from build123d import *

# Parameters (mm, degrees)
SKETCH1_R           = 69.85
BOSS_EXTRUDE1_DEPTH = 6.35
SKETCH4_R           = 0.59055
CUT_EXTRUDE1_DEPTH  = 49.26
CUT_EXTRUDE2_START  = -51.8
SKETCH6_R           = 0.59055
CUT_EXTRUDE2_DEPTH  = 77.349261314
LOX_START           = -7.35
SKETCH7_R           = 0.8255
LOX_HOLES_DEPTH     = 8.35
CIRPATTERN1_COUNT   = 18
SKETCH8_R           = 3.2639
CUT_EXTRUDE4_DEPTH  = 7.35
CIRPATTERN2_COUNT   = 12


with BuildPart() as part:
    # Sketch1 → Boss-Extrude1 (new body)
    with BuildSketch(Plane(origin=(0, 0, 0), x_dir=(1, 0, 0), z_dir=(0, 1, 0))):
        Circle(SKETCH1_R)
    extrude(amount=BOSS_EXTRUDE1_DEPTH)

    # Sketch4 → Cut-Extrude1 (cut, through all)
    with BuildSketch(Plane(origin=(-3.917869343, -6.785948759, 0), x_dir=(-0.866025404, 0.5, 0), z_dir=(0.5, 0.866025404, 0))):
        with Locations((-4.52396584, 0)):
            Circle(SKETCH4_R)
    cut_extrude1 = extrude(amount=CUT_EXTRUDE1_DEPTH, mode=Mode.SUBTRACT)

    # Sketch6 → Cut-Extrude2 (cut)
    with BuildSketch(Plane(origin=(5.187869343, -8.985653285, 0), x_dir=(0.866025404, 0.5, 0), z_dir=(0.5, -0.866025404, 0)).offset(CUT_EXTRUDE2_START)):
        with Locations((30.67130657, 0)):
            Circle(SKETCH6_R)
    cut_extrude2 = extrude(amount=CUT_EXTRUDE2_DEPTH, mode=Mode.SUBTRACT)

    # Sketch7 → LOx Holes (cut)
    with BuildSketch(Plane(origin=(0, 6.35, 0), x_dir=(1, 0, 0), z_dir=(0, 1, 0)).offset(LOX_START)):
        with Locations((24.13, 0)):
            Circle(SKETCH7_R)
        with Locations((16.51, 0)):
            Circle(SKETCH7_R)
    lox_holes = extrude(amount=LOX_HOLES_DEPTH, mode=Mode.SUBTRACT)

    # CirPattern1: Cut-Extrude1, Cut-Extrude2, LOx Holes ×18 about axis
    cirpattern1_axis = Axis((0, 0, 0), (0, 1, 0))
    for i in range(1, CIRPATTERN1_COUNT):
        add(cut_extrude1.rotate(cirpattern1_axis, i * 360 / CIRPATTERN1_COUNT), mode=Mode.SUBTRACT)
        add(cut_extrude2.rotate(cirpattern1_axis, i * 360 / CIRPATTERN1_COUNT), mode=Mode.SUBTRACT)
        add(lox_holes.rotate(cirpattern1_axis, i * 360 / CIRPATTERN1_COUNT), mode=Mode.SUBTRACT)

    # Sketch8 → Cut-Extrude4 (cut, through all)
    with BuildSketch(Plane.XZ):
        with Locations((-60.96, 0)):
            Circle(SKETCH8_R)
    cut_extrude4 = extrude(amount=-CUT_EXTRUDE4_DEPTH, mode=Mode.SUBTRACT)

    # CirPattern2: Cut-Extrude4 ×12 about axis
    cirpattern2_axis = Axis((0, 0, 0), (0, 1, 0))
    for i in range(1, CIRPATTERN2_COUNT):
        add(cut_extrude4.rotate(cirpattern2_axis, i * 360 / CIRPATTERN2_COUNT), mode=Mode.SUBTRACT)


solid = part.part
Build history of the part. All positions in model axes, mm. Coordinates: 2 decimals unless noted, no trailing zeros. Order: outer loops, then holes, each group sorted by start corner. A loop starts at its lowest first (then second) coordinate and runs counter-clockwise, first axis right, second up. Notation, with made-up numbers: (79.25, -28.75) - (129.25, -28.75) arc R20 ccw to (129.25, 7.25) - close; hole circle Ø4 at (46, 1.5). An arc over 180 degrees is marked (long way). Put each result on its own line as item: value.
1. Saw through at A-A (z = -60.96). Write the cut outline in (x, y).
Answer sheet:
outline: (-34.1, 0) - (-3.26, 0) - (-3.26, 6.35) - (-34.1, 6.35) - close; (3.26, 0) - (34.1, 0) - (34.1, 6.35) - (3.26, 6.35) - close
2. Pull direction Y, two halves, no side cores. Call faces 1 (the face through (-5.065, 3.102, -5.014)), 2 (the face through (-16.5, 2.94, -28.62)), 3 (the face through (-30.055, 3.131, 49.557)): pulls with the +Y half, pulls with the -Y half, needs draft (parallel to the pull), parting line crosses it, or undercut.
Answer sheet:
face 1: undercut
face 2: undercut
face 3: needs draft
3. Saw through at C-C (z = 53). Write the cut outline in (x, y), and give its area (3 significant figures).
Answer sheet:
outline: (-45.5, 0) - (-33.74, 0) - (-33.74, 6.35) - (-45.5, 6.35) - close; (-27.22, 0) - (27.22, 0) - (27.22, 6.35) - (-27.22, 6.35) - close; (33.74, 0) - (45.5, 0) - (45.5, 6.35) - (33.74, 6.35) - close
area: 495 mm^2
4. Saw through at D-D (y = 3). Give the number of separate pieces and of enclosed holes in the cut face, and give its area (3 significant figures).
Answer sheet:
separate pieces: 1
enclosed holes: 84
area: 14,800 mm^2
5. Drop flat-ended pins along their axis: P1, Ø3, axis at y = 3.5, z = 31.5, coming from the +X side; P2, Ø3, axis at x = -46.5, y = 4, coming from the -Z side; P3, Ø1, axis at y = 2, z = -11.5, coming from the +X side. Give the stop position or say it passes through.
Answer sheet:
P1: stops at x = 63.08
P2: stops at z = -53.42
P3: stops at x = 68.98
6. Probe line 1 along X through (y, z) = (4.5, -8.5); line 2 along Z through (x, y) = (-18, 1.5); line 3 along X through (y, z) = (5.5, 21). List the from-to ranges inside material, lowest first. Write a range as [from, to].
Answer sheet:
line 1: x = [-69.33, -23.46], [-21.89, 21.89], [23.46, 69.33]
line 2: z = [-67.49, -16.18], [-14.84, 14.84], [16.18, 67.49]
line 3: x = [-66.62, -25.31], [-24.16, -12.88], [-11.25, 11.25], [12.88, 24.16], [25.31, 66.62]
7. Saw through at B-B (x = 53.5). Write the cut outline in (y, z), and give its area (3 significant figures).
Answer sheet:
outline: (0, -44.91) - (6.35, -44.91) - (6.35, -33.67) - (0, -33.67) - close; (0, -27.29) - (6.35, -27.29) - (6.35, 27.29) - (0, 27.29) - close; (0, 33.67) - (6.35, 33.67) - (6.35, 44.91) - (0, 44.91) - close
area: 489 mm^2
